Study the drawing (mm; zero at the part's minimum x, y, z) and answer. A direction names the side the tool comes from. Coordinates: 2 decimals unless noted, no trailing zeros. Write each loop counter-clockwise with the first axis right and the second up, starting at its lowest first coordinate (ties: lowest second). Pieces come first, ordered by that corner, then holes. Notation, with made-up numbers: (27, 27) - (85, 27) arc R18 ccw to (85, 33) - close; hole circle Ø10 at (-30, -18). An arc over 180 degrees is marked (long way). One line per item, written item: value.
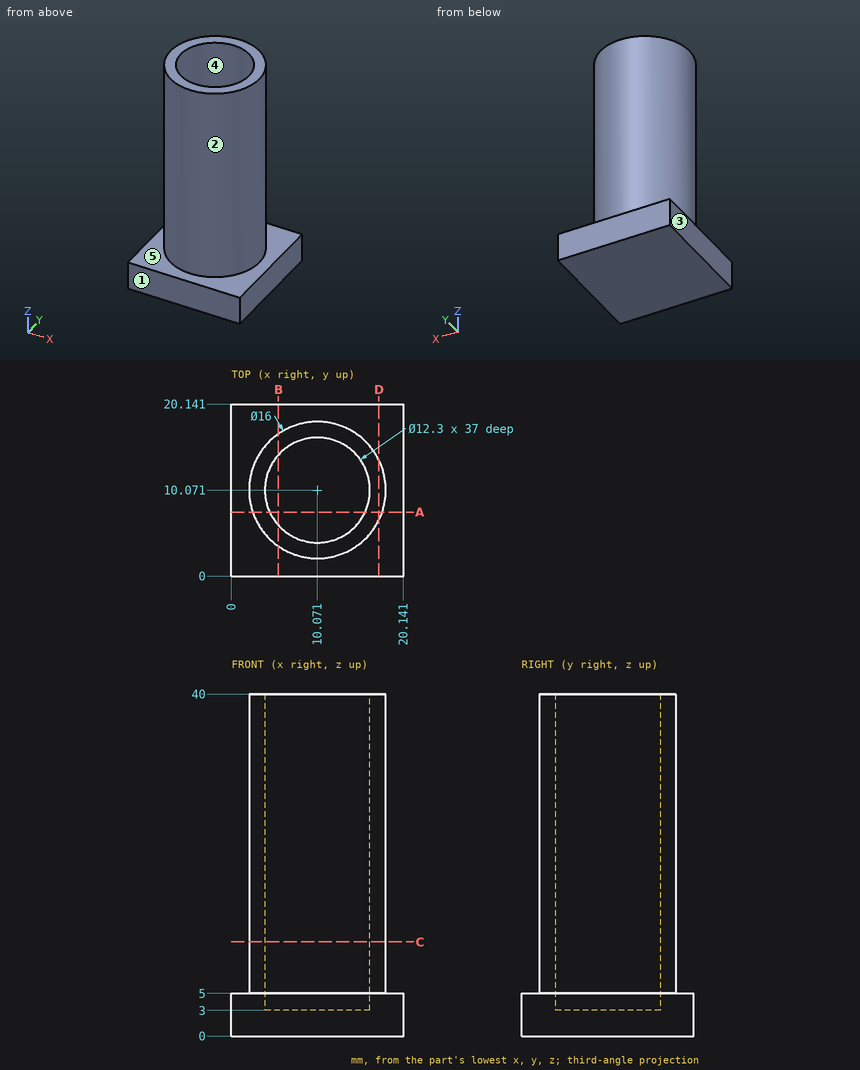
Item 1: Consider probe 1 along Z at (x, y) = (13, 10); probe 2 along Y at (x, z) = (10.5, 36) (1 decimal); probe 3 along X at (y, z) = (10.25, 29.5). Determine where each line is inside the solid, lowest interval first.
Evaluation:
probe 1: z = 0 to 3
probe 2: y = 2.1 to 3.9, 16.2 to 18.1
probe 3: x = 2.07 to 3.92, 16.22 to 18.07
Item 2: Determine the mould class of the marked faces 3, 4 and 5 for opening direction X: +X half, -X half, draft (parallel to the pull), parting line (faces both ways), or undercut.
Evaluation:
face 3: -X half
face 4: undercut
face 5: draft
Item 3: Which of the six approach directions +Z, -Z, +X, -X, +Y, -Y give full straight-line access (tool end or side, diameter ignored) to the marked faces 1 and 2?
Evaluation:
face 1: +Z, -Z, +X, -X, -Y
face 2: +Z
Item 4: Given pin 1 (3 mm diameter, centred on x = 3.5, z = 13, fed in from +Y); pin 2 (3 mm diameter, centred on x = 12.5, z = 11.5, fed in from +Y); pin 3 (12 mm diameter, centred on y = 3.5, z = 13, fed in from -X), each flat-ended and moving along its own axis, determine where each tip first touches the part or whether it passes through.
Evaluation:
pin 1: stops at y = 16.26
pin 2: stops at y = 18.02
pin 3: stops at x = 2.09
Item 5: Section A-A, the plane y = 7.5 is taken. Determine the outline of the cut face in (x, z) (1 decimal).
Evaluation:
outline: (0, 0) - (20.1, 0) - (20.1, 5) - (17.6, 5) - (17.6, 40) - (15.7, 40) - (15.7, 3) - (4.5, 3) - (4.5, 40) - (2.5, 40) - (2.5, 5) - (0, 5) - close
Item 6: Section C-C, the plane z = 11 is taken. Determine the outline of the cut face in (x, y).
Evaluation:
outline: circle Ø16 at (10.07, 10.07); hole circle Ø12.3 at (10.07, 10.07)
Item 7: Section B-B, the plane x = 5.5 is taken. Determine the outline of the cut face in (y, z) (1 decimal), then the cut area to 3 significant figures.
Evaluation:
outline: (0, 0) - (20.1, 0) - (20.1, 5) - (16.6, 5) - (16.6, 40) - (14.2, 40) - (14.2, 3) - (6, 3) - (6, 40) - (3.5, 40) - (3.5, 5) - (0, 5) - close
area: 256 mm2
Item 8: Section D-D, the plane x = 17.25 is taken. Determine the outline of the cut face in (y, z), then the cut area to 3 significant figures.
Evaluation:
outline: (0, 0) - (20.14, 0) - (20.14, 5) - (13.6, 5) - (13.6, 40) - (6.54, 40) - (6.54, 5) - (0, 5) - close
area: 348 mm2
